Check sheet for the modelled part. Datum: model origin and axes. Units: mm. Face numbers are marked on the shaded views. A direction names the side the tool comes from. Round coordinates to 2 decimals unless told otherwise and drop trailing zeros. Write each loop counter-clockwise with the first axis right and the second up, starting at its lowest first coordinate (ties: lowest second). Pieces come first, ordered by that corner, then holes. Notation, with made-up numbers: (60, 10) -> (108, 10) arc R9 ccw to (108, 18) -> close; hole circle Ø3 at (-19.75, 69). An arc over 180 degrees is marked (long way). One line per item, written item: value. Start each with the question number.
```python
from build123d import *

# Parameters (mm, degrees)
SMUSSO2_SIZE             = 0.5
SMUSSO2_SIZE2            = 0.431608995
SCHIZZO6_R               = 5.5
TAGLIO_ESTRUSIONE1_DEPTH = 21.738887755


with BuildPart() as part:
    # Schizzo1 → Rivoluzione1 (revolve)
    with BuildSketch(Plane.XY):
        Polygon((0, -14.8), (-7.75, -14.8), (-10.359639314, 0), (0, 0), align=None)
    revolve(axis=Axis((0, 0, 0), (0, -1, 0)))

    # Schizzo2 → Taglia-Rivoluzione1 (revolve, cut)
    with BuildSketch(Plane.XY):
        Polygon((-9.824143265, -3.03694901), (-8.16966624, -2.745220072), (-7.683451342, -5.50268178), (-9.337928368, -5.794410718), align=None)
        Polygon((-8.824143265, -8.70823083), (-8.337928368, -11.465692538), (-6.683451342, -11.1739636), (-7.16966624, -8.416501891), align=None)
    revolve(axis=Axis((0, 0, 0), (0, -1, 0)), mode=Mode.SUBTRACT)

    # Smusso2
    smusso2_edges = [part.edges().sort_by_distance(p)[0] for p in [
        (10.359639314, 0, 0),
    ]]
    smusso2_side = [part.faces().sort_by_distance(p)[0] for p in [
        (10.09189129, -1.518474505, 0),
    ]]
    chamfer(smusso2_edges, length=SMUSSO2_SIZE, length2=SMUSSO2_SIZE2, reference=smusso2_side[0])

    # Schizzo6 → Taglio-Estrusione1 (cut, through all)
    with BuildSketch(Plane.XZ.offset(14.8)):
        Circle(SCHIZZO6_R)
    extrude(amount=-TAGLIO_ESTRUSIONE1_DEPTH, mode=Mode.SUBTRACT)


solid = part.part
```
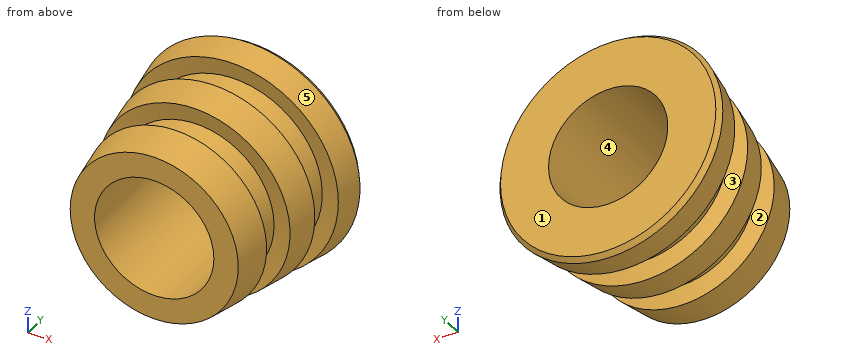
1. Cross-section at D-D (y = -12.25). Record the cut outline in (x, z), plus the area to 3 significant figures.
2. Material ranges on probe 1 along X at (y, z) = (-9.5, 1.25); probe 2 along X at (y, z) = (-8.25, -1.25); probe 3 along Y at (x, z) = (3.75, 7.5), recorded low to high.
3. Cross-section at A-A (z = 0). Record the cut outline in (x, y), plus the area to 3 significant figures.
4. Cross-section at C-C (y = -7.25). Record the cut outline in (x, z), plus the area to 3 significant figures.
5. Depth check by flat-ended pin: pin 1 Ø2 at (y, z) = (-8, 1.5) entering from +X; pin 2 Ø1 at (y, z) = (-9.5, -6.5) entering from -X; pin 3 Ø2 at (y, z) = (-10, -4.5) entering from +X. Enter the tip coordinate at first touch or a pass-through.
6. Release check for a two-part mould opening along Y. For the marked faces 3, 4 and 5 record: +Y half, -Y half, draft (parallel to the pull), parting line (faces both ways), or undercut.
7. Access from +Z, -Z, +X, -X, +Y, -Y to the whole of each face (thin tool, end or side, straight path). Record for the marked faces 1 and 2.
8. Cross-section at B-B (x = 0). Record the cut outline in (y, z).
Working result:
1. outline: circle Ø16.4 at (0, 0); hole circle Ø11 at (0, 0)
1. area: 116 mm^2
2. probe 1: x = -6.87 to -5.36, 5.36 to 6.87
2. probe 2: x = -8.82 to -5.36, 5.36 to 8.82
2. probe 3: y = -8.63 to -5.63, -2.78 to 0
3. outline: (-10.27, -0.49) -> (-9.82, -3.04) -> (-8.17, -2.75) -> (-7.68, -5.5) -> (-9.34, -5.79) -> (-8.82, -8.71) -> (-7.17, -8.42) -> (-6.68, -11.17) -> (-8.34, -11.47) -> (-7.75, -14.8) -> (-5.5, -14.8) -> (-5.5, 0) -> (-9.93, 0) -> close; (5.5, -14.8) -> (7.75, -14.8) -> (8.34, -11.47) -> (6.68, -11.17) -> (7.17, -8.42) -> (8.82, -8.71) -> (9.34, -5.79) -> (7.68, -5.5) -> (8.17, -2.75) -> (9.82, -3.04) -> (10.27, -0.49) -> (9.93, 0) -> (5.5, 0) -> close
3. area: 86.2 mm^2
4. outline: circle Ø18.16 at (0, 0); hole circle Ø11 at (0, 0)
4. area: 164 mm^2
5. pin 1: stops at x = 9.05
5. pin 2: stops at x = -3.58
5. pin 3: stops at x = 5.97
6. face 3: undercut
6. face 4: draft
6. face 5: -Y half
7. face 1: +Z, -Z, +X, -X, +Y
7. face 2: none
8. outline: (-14.8, -7.75) -> (-11.47, -8.34) -> (-11.17, -6.68) -> (-8.42, -7.17) -> (-8.71, -8.82) -> (-5.79, -9.34) -> (-5.5, -7.68) -> (-2.75, -8.17) -> (-3.04, -9.82) -> (-0.49, -10.27) -> (0, -9.93) -> (0, -5.5) -> (-14.8, -5.5) -> close; (-14.8, 5.5) -> (0, 5.5) -> (0, 9.93) -> (-0.49, 10.27) -> (-3.04, 9.82) -> (-2.75, 8.17) -> (-5.5, 7.68) -> (-5.79, 9.34) -> (-8.71, 8.82) -> (-8.42, 7.17) -> (-11.17, 6.68) -> (-11.47, 8.34) -> (-14.8, 7.75) -> close
